from build123d import *

# Parameters (mm, degrees)
SKETCH1_R           = 3.137422597
BOSS_EXTRUDE1_DEPTH = 4.572
FILLET3_R           = 0.254
SKETCH2_R           = 4.111492789
BOSS_EXTRUDE3_DEPTH = 0.762


with BuildPart() as part:
    # Sketch1 → Boss-Extrude1 (new body)
    with BuildSketch(Plane(origin=(0, 0, 0), x_dir=(1, 0, 0), z_dir=(0, 1, 0))):
        Circle(SKETCH1_R)
    extrude(amount=BOSS_EXTRUDE1_DEPTH)

    # Fillet3
    fillet3_edges = [part.edges().sort_by_distance(p)[0] for p in [
        (-3.137422597, 0, 0),
    ]]
    fillet(fillet3_edges, radius=FILLET3_R)

    # Sketch2 → Boss-Extrude3 (add)
    with BuildSketch(Plane(origin=(0, 4.572, 0), x_dir=(1, 0, 0), z_dir=(0, 1, 0))):
        Circle(SKETCH2_R)
    extrude(amount=BOSS_EXTRUDE3_DEPTH)


solid = part.part
Build history of the part. All positions in model axes, mm. A direction names the side the tool comes from. Coordinates: 2 decimals unless noted, no trailing zeros. Order: outer loops, then holes, each group sorted by start corner. A loop starts at its lowest first (then second) coordinate and runs counter-clockwise, first axis right, second up. Notation, with made-up numbers: (84, 9) - (113, 9) arc R36 cw to (113, 47) - close; hole circle Ø6 at (18.25, 18.25). An arc over 180 degrees is marked (long way). Put each result on its own line as item: value.
1. Tool access for faces 1 (the face through (0, 5.334, 0)), 2 (the face through (-3, 4.572, 2)): list every direction of +Z, -Z, +X, -X, +Y, -Y with a clear straight run to the whole face (end or side of a thin tool).
Answer sheet:
face 1: +Z, -Z, +X, -X, +Y
face 2: -Y
2. Probe line 1 along Y through (x, z) = (3.75, -0.75); line 2 along Z through (x, y) = (0, 0.7); line 3 along Y through (x, z) = (2.5, 1.5). List the from-to ranges inside material, lowest first. Write a range as [from, to].
Answer sheet:
line 1: y = [4.57, 5.33]
line 2: z = [-3.14, 3.14]
line 3: y = [0, 5.33]
3. Saw through at A-A (x = 0). Write the cut outline in (y, z).
Answer sheet:
outline: (0, -2.88) arc R0.25 ccw to (0.25, -3.14) - (4.57, -3.14) - (4.57, -4.11) - (5.33, -4.11) - (5.33, 4.11) - (4.57, 4.11) - (4.57, 3.14) - (0.25, 3.14) arc R0.25 ccw to (0, 2.88) - close
4. Saw through at C-C (y = 1.95). Write the cut outline in (x, z), and give its area (3 significant figures).
Answer sheet:
outline: circle Ø6.27 at (0, 0)
area: 30.9 mm^2
5. Saw through at B-B (z = 0). Write the cut outline in (x, y), and give its area (3 significant figures).
Answer sheet:
outline: (-4.11, 4.57) - (-3.14, 4.57) - (-3.14, 0.25) arc R0.25 ccw to (-2.88, 0) - (2.88, 0) arc R0.25 ccw to (3.14, 0.25) - (3.14, 4.57) - (4.11, 4.57) - (4.11, 5.33) - (-4.11, 5.33) - close
area: 34.9 mm^2
6. Drop flat-ended pins along their axis: P1, Ø1, axis at y = 4.5, z = 0, coming from the -X side; P2, Ø1, axis at x = 1.5, y = 3, coming from the -Z side. Give the stop position or say it passes through.
Answer sheet:
P1: stops at x = -4.11
P2: stops at z = -2.97
7. Saw through at D-D (x = -3.25). Write the cut outline in (y, z), and give its area (3 significant figures).
Answer sheet:
outline: (4.57, -2.52) - (5.33, -2.52) - (5.33, 2.52) - (4.57, 2.52) - close
area: 3.84 mm^2
